```python
from build123d import *

# Parameters (mm, degrees)
SKETCH_1_W                  = 23
SKETCH_1_H                  = 17
EXTRUDE_1_DEPTH             = 6.5
SKETCH_2_W                  = 20
SKETCH_2_H                  = 15.5
CUT_EXTRUDE_1_DEPTH         = 5
SKETCH_3_W                  = 23
SKETCH_3_H                  = 1.5
EXTRUDE_2_DEPTH             = 12.6
EXTRUDE_3_DEPTH             = 3
EXTRUDE_6_REACH             = 21.397
SKETCH_7_W                  = 1.5
SKETCH_7_H                  = 7.259859141
EXTRUDE_6_DIRECTION_2_REACH = 21.397
HOLE_WIZARD_M3_1_D          = 3.2
FILLET_1_R                  = 3


with BuildPart() as part:
    # 草图1 → 凸台-拉伸1 (new body)
    with BuildSketch(Plane.XY):
        Rectangle(SKETCH_1_W, SKETCH_1_H)
    extrude(amount=EXTRUDE_1_DEPTH)

    # 草图2 → 切除-拉伸1 (cut)
    with BuildSketch(Plane.XY.offset(6.5)):
        with Locations((0, -0.75)):
            Rectangle(SKETCH_2_W, SKETCH_2_H)
    extrude(amount=-CUT_EXTRUDE_1_DEPTH, mode=Mode.SUBTRACT)

    # 草图3 → 凸台-拉伸2 (add)
    with BuildSketch(Plane(origin=(0, 0, 0), x_dir=(-1, 0, 0), z_dir=(0, 0, -1))):
        with Locations((0, -7.75)):
            Rectangle(SKETCH_3_W, SKETCH_3_H)
    extrude(amount=EXTRUDE_2_DEPTH)

    # 草图4 → 凸台-拉伸3 (add)
    with BuildSketch(Plane(origin=(0, -7, 0), x_dir=(1, 0, 0), z_dir=(0, 1, 0))):
        Polygon((4.965212315, 6.3), (2.482606158, 10.6), (-2.482606158, 10.6), (-4.965212315, 6.3), (-2.482606158, 2), (2.482606158, 2), align=None)
        Polygon((3.233161507, 6.3), (1.616580754, 9.1), (-1.616580754, 9.1), (-3.233161507, 6.3), (-1.616580754, 3.5), (1.616580754, 3.5), align=None, mode=Mode.SUBTRACT)
    extrude(amount=EXTRUDE_3_DEPTH)

    # 凸台-拉伸6: up to this face of the body (flat: up to its plane)
    extrude_6_end = Plane(part.part.faces().sort_by_distance((0, -7, -6.3))[0])
    # 草图7 → 凸台-拉伸6 (add, up to the picked face)
    with BuildSketch(Plane(origin=(0, -3.5, -3.5), x_dir=(-1, 0, 0), z_dir=(0, -0.7071067811865475, -0.7071067811865477)), mode=Mode.PRIVATE) as extrude_6_sk1:
        with Locations((-10.75, -1.319817897)):
            Rectangle(SKETCH_7_W, SKETCH_7_H)
    extrude_6_tool1 = split(extrude(extrude_6_sk1.sketch, amount=EXTRUDE_6_REACH, mode=Mode.PRIVATE), bisect_by=extrude_6_end, keep=Keep.BOTH, mode=Mode.PRIVATE)
    extrude_6 = extrude_6_tool1.solids().sort_by(Axis((10.75, -4.433252, -2.566748), (0, -0.7071067811865475, -0.7071067811865477)))[0]
    add(extrude_6)

    # 凸台-拉伸6 direction 2: up to this face of the body (flat: up to its plane)
    extrude_6_direction_2_end = Plane(part.part.faces().sort_by_distance((0, 0.75, 0))[0])
    # 草图7 → 凸台-拉伸6 direction 2 (add, up to the picked face)
    with BuildSketch(Plane(origin=(0, -3.5, -3.5), x_dir=(-1, 0, 0), z_dir=(0, -0.7071067811865475, -0.7071067811865477)), mode=Mode.PRIVATE) as extrude_6_direction_2_sk1:
        with Locations((-10.75, -1.319817897)):
            Rectangle(SKETCH_7_W, SKETCH_7_H)
    extrude_6_direction_2_tool1 = split(extrude(extrude_6_direction_2_sk1.sketch, amount=-EXTRUDE_6_DIRECTION_2_REACH, mode=Mode.PRIVATE), bisect_by=extrude_6_direction_2_end, keep=Keep.BOTH, mode=Mode.PRIVATE)
    extrude_6_direction_2 = extrude_6_direction_2_tool1.solids().sort_by(Axis((10.75, -4.433252, -2.566748), (0, 0.7071067811865475, 0.7071067811865477)))[0]
    add(extrude_6_direction_2)

    # 镜向1: 凸台-拉伸6, 凸台-拉伸6 direction 2 across plane
    add(extrude_6.mirror(Plane(origin=(0, 0, 0), x_dir=(0, 0, 1), z_dir=(1, 0, 0))))
    add(extrude_6_direction_2.mirror(Plane(origin=(0, 0, 0), x_dir=(0, 0, 1), z_dir=(1, 0, 0))))

    # M3 间隙孔1 (through all)
    with Locations(Plane(origin=(0, -7, 0), x_dir=(1, 0, 0), z_dir=(0, 1, 0))):
        with Locations((0, 6.3)):
            Hole(HOLE_WIZARD_M3_1_D / 2)

    # 圆角1
    fillet_1_edges = [part.edges().sort_by_distance(p)[0] for p in [
        (-11.5, -7.75, -12.6),
        (11.5, -7.75, -12.6),
    ]]
    fillet(fillet_1_edges, radius=FILLET_1_R)


solid = part.part
```
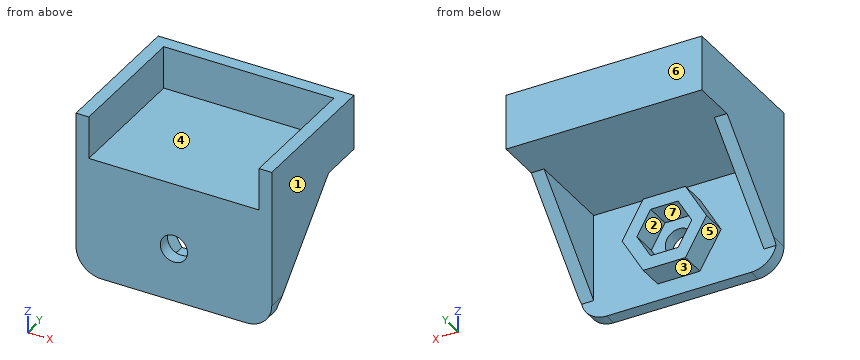
Here's how the part is built. I have some questions about the finished solid (model axes, mm). Face numbers are marked on the shaded views. A direction names the side the tool comes from. Round coordinates to 2 decimals unless told otherwise and drop trailing zeros. Loops run counter-clockwise (first coordinate to the right, second up) from the corner with the lowest first, then second, coordinate; pieces in that order, holes last.
1. Suppose I cut it at C-C, the plane z = -5.25. Please give me the cut outline in (x, y).
Answers:
outline: (-11.5, -8.5) - (-1.21, -8.5) - (-1.21, -7) - (-2.63, -7) - (-2.63, -4) - (-4.36, -4) - (-4.36, -7) - (-10, -7) - (-10, -1.98) - (-11.5, -1.98) - close; (1.21, -8.5) - (11.5, -8.5) - (11.5, -1.98) - (10, -1.98) - (10, -7) - (4.36, -7) - (4.36, -4) - (2.63, -4) - (2.63, -7) - (1.21, -7) - close
2. Thinking about a two-plate mould opening in Z: for the marked faces 1, 2 and 3, which applies, released by +Z, released by -Z, zero draft, split by the parting line, or undercut?
Answers:
face 1: zero draft
face 2: undercut
face 3: released by -Z
3. Suppose I cut it at B-B, the plane y = -5. Please give me the cut outline in (x, z).
Answers:
outline: (-11.5, -8.27) - (-10, -8.27) - (-10, 0) - (10, 0) - (10, -8.27) - (11.5, -8.27) - (11.5, 6.5) - (10, 6.5) - (10, 1.5) - (-10, 1.5) - (-10, 6.5) - (-11.5, 6.5) - close; (-4.97, -6.3) - (-2.48, -10.6) - (2.48, -10.6) - (4.97, -6.3) - (2.48, -2) - (-2.48, -2) - close; hole (-3.23, -6.3) - (-1.62, -9.1) - (1.62, -9.1) - (3.23, -6.3) - (1.62, -3.5) - (-1.62, -3.5) - close
4. If I drill on probe 1 along Z at (x, y) = (0, -7.5); probe 2 along X at (y, z) = (5.5, 3.5); probe 3 along X at (y, z) = (-6.75, -9), over which ranges is the centre line in solid material (lowest first)?
Answers:
probe 1: z = -12.6 to -7.9, -4.7 to 1.5
probe 2: x = -11.5 to -10, 10 to 11.5
probe 3: x = -11.5 to -10, -3.41 to -1.67, 1.67 to 3.41, 10 to 11.5
5. Suppose I cut it at A-A, the plane x = 0. Please give me the cut outline in (y, z), and give its area (3 significant figures).
Answers:
outline: (-8.5, -12.6) - (-7, -12.6) - (-7, -10.6) - (-4, -10.6) - (-4, -9.1) - (-7, -9.1) - (-7, -7.9) - (-8.5, -7.9) - close; (-8.5, -4.7) - (-7, -4.7) - (-7, -3.5) - (-4, -3.5) - (-4, -2) - (-7, -2) - (-7, 0) - (8.5, 0) - (8.5, 6.5) - (7, 6.5) - (7, 1.5) - (-8.5, 1.5) - close
area: 56.1 mm2
6. Will these pins go through, and if not, where does the flat tip stop? pin 1 (1.5 mm diameter, centred on x = -0.5, y = -6, fed in from -Z); pin 2 (3 mm diameter, centred on x = -2, z = -10, fed in from +Y); pin 3 (0.9 mm diameter, centred on x = 0, y = -5.5, fed in from +Z).
Answers:
pin 1: stops at z = -10.6
pin 2: stops at y = -4
pin 3: stops at z = 1.5
7. For the marked faces 4, 5, 6 and 7, which set-ups out of +Z, -Z, +X, -X, +Y, -Y let a thin tool reach every point of the face, with its end or its side?
Answers:
face 4: +Z, -Y
face 5: -Z, +Y
face 6: +Z, -Z, +X, -X, +Y
face 7: +Y
8. Suppose I cut it at D-D, the plane y = 5.5. Please give me the cut outline in (x, z).
Answers:
outline: (-11.5, 0) - (11.5, 0) - (11.5, 6.5) - (10, 6.5) - (10, 1.5) - (-10, 1.5) - (-10, 6.5) - (-11.5, 6.5) - close
